from build123d import *

# Parameters (mm, degrees)
F0_W     = 135.9543129802
F0_H     = 70.837918669
F1_DEPTH = 25.4
F2_W     = 135.9543129802
F2_H     = 73.7939976811
F2_H_2   = 25.4
F3_DEPTH = 9.525
F4_W     = 15.9723907709
F4_H     = 70.837918669
F5_DEPTH = 57.912
F7_DEPTH = 25.4


with BuildPart() as f1:
    # F0 (on Front) → F1 (new body)
    with BuildSketch(Plane.XZ):
        with Locations((16.0006545484, -2.0842719823)):
            Rectangle(F0_W, F0_H)
    extrude(amount=F1_DEPTH)

    # F2 (on face) → F3 (join)
    with BuildSketch(Plane.XY.offset(33.3346873522)):
        with Locations((16.0006545484, -62.2969988406)):
            Rectangle(F2_W, F2_H)
        with Locations((16.0006545484, -12.7)):
            Rectangle(F2_W, F2_H_2)
    extrude(amount=F3_DEPTH)

    # F4 (on face) → F5 (join)
    with BuildSketch(Plane.XZ.offset(25.4)):
        with Locations((18.005028367, -2.0842719823)):
            Rectangle(F4_W, F4_H)
    extrude(amount=F5_DEPTH)

    # F6 (on face) → F7 (cut)
    with BuildSketch(Plane.YZ.offset(25.9912237525)):
        with BuildLine():
            Line((-83.312, -37.5032313168), (-41.5840882454, -37.5032313168))
            ThreePointArc((-41.5840882454, -37.5032313168), (-57.0724279587, -7.8575184678), (-83.312, 12.8847527793))
            Line((-83.312, 12.8847527793), (-83.312, -37.5032313168))
        make_face()
    extrude(amount=-F7_DEPTH, mode=Mode.SUBTRACT)


solid = f1.part
Geometry check sheet. Reference: the model listing, model coordinates, mm. A direction names the side the tool comes from. Give positions to 0.01 mm unless a question says otherwise; leave off trailing zeros. Loops run counter-clockwise (first coordinate to the right, second up) from the corner with the lowest first, then second, coordinate; pieces in that order, holes last.
(1) Section check B-B on x = 48. Record the cut outline in (y, z).
From the geometry:
outline: (-99.19, 33.33) - (-25.4, 33.33) - (-25.4, -37.5) - (0, -37.5) - (0, 42.86) - (-99.19, 42.86) - close
(2) Section check D-D on y = -86.5. Record the cut outline in (x, z), then the cut area to 3 significant figures.
From the geometry:
outline: (-51.98, 33.33) - (83.98, 33.33) - (83.98, 42.86) - (-51.98, 42.86) - close
area: 1,290 mm2
(3) Set-up check for faces 1 (the flat face through (0, -62, 33.335)), 2 (the flat face through (18, -83.312, 23)), 3 (the flat face through (10.019, -48, 5)), 4 (the flat face through (55, -25.4, -2)), 5 (the flat face through (15, -16, -37.503)): record each of +Z, -Z, +X, -X, +Y, -Y from which the full face is reachable in a straight line by a thin tool's end or side.
From the geometry:
face 1: -Z, -Y
face 2: -Z, +X, -X, -Y
face 3: -Z, -X, -Y
face 4: -Z, +X, -Y
face 5: -Z, +X, -X, +Y, -Y
(4) Depth check by flat-ended pin: pin 1 Ø4 at (y, z) = (-34.5, 17) entering from -X; pin 2 Ø5 at (x, z) = (16, 25.5) entering from -Y; pin 3 Ø8 at (x, z) = (-8.5, 10.5) entering from -Y. Enter the tip coordinate at first touch or a pass-through.
From the geometry:
pin 1: stops at x = 10.02
pin 2: stops at y = -83.31
pin 3: stops at y = -25.4
(5) Section check C-C on z = 24. Record the cut outline in (x, y), then the cut area to 3 significant figures.
From the geometry:
outline: (-51.98, -25.4) - (10.02, -25.4) - (10.02, -83.31) - (25.99, -83.31) - (25.99, -25.4) - (83.98, -25.4) - (83.98, 0) - (-51.98, 0) - close
area: 4,380 mm2
(6) Section check A-A on y = -33.5. Record the cut outline in (x, z).
From the geometry:
outline: (-51.98, 33.33) - (10.02, 33.33) - (10.02, -37.5) - (25.99, -37.5) - (25.99, 33.33) - (83.98, 33.33) - (83.98, 42.86) - (-51.98, 42.86) - close
(7) Thickness scan on L1, parallel to Z at x = 42, y = -49.5; L2, parallel to X at y = -61.5, z = 22; L3, parallel to Y at x = -16, z = -24. Record the ranges inside material, lowest first.
From the geometry:
L1: z = 33.33 to 42.86
L2: x = 10.02 to 25.99
L3: y = -25.4 to 0
